Autodesk Inventor part; units mm, degrees
ref_plane "FOR_PIN_1_XY" through (0, 2, 0) normal (0, 1, 0) x (1, 0, 0)
ref_plane "FOR_PIN_1_YZ" through (0, 2, 0) normal (1, 0, 0) x (0, 0, -1)
ref_plane "FOR_PIN_1_ZX" through (0, 2, 0) normal (0, 0, -1) x (0, 1, 0)
sketch "Sketch_2" plane through (0, 0, 0) normal (0, 1, 0) x (-1, 0, 0)
  line L0 (1, -0.402) -> (1, 0.402)
  line L1 (1, 0.402) -> (0.7211, 1)
  line L2 (0.7211, 1) -> (-0.7211, 1)
  line L3 (-0.7211, 1) -> (-1, 0.402)
  line L4 (-1, 0.402) -> (-1, -0.402)
  line L5 (-1, -0.402) -> (-0.7211, -1)
  line L6 (-0.7211, -1) -> (0.7211, -1)
  line L7 (0.7211, -1) -> (1, -0.402)
extrude "Extrusion1" add sketch "Sketch_2" along normal blind 2
pattern_linear "Rectangular Pattern1" count 6 spacing 2 along (1, 0, 0) of "Extrusion1"
sketch "Sketch_6" plane through (-1, 0, 0) normal (1, 0, 0) x (0, 0, -1)
  line L0 (-0.75, 0.5) -> (-0.75, 0)
  line L1 (-0.75, 0) -> (0.75, 0)
  line L2 (0.75, 0) -> (0.75, 0.5)
  line L3 (0.75, 0.5) -> (-0.75, 0.5)
extrude "Extrusion2" cut sketch "Sketch_6" along normal blind 12
sketch "Sketch_4" plane through (0, 0, 0) normal (0, 1, 0) x (-1, 0, 0)
  line L0 (0.25, -0.25) -> (0.25, 0.25)
  line L1 (0.25, 0.25) -> (-0.25, 0.25)
  line L2 (-0.25, 0.25) -> (-0.25, -0.25)
  line L3 (-0.25, -0.25) -> (0.25, -0.25)
extrude "Extrusion3" cut sketch "Sketch_4" along normal blind 2
pattern_linear "Rectangular Pattern2" count 6 spacing 2 along (1, 0, 0) of "Extrusion3"
sketch "Sketch_9" plane through (0, 0, 0) normal (0, 0, 1) x (1, 0, 0)
  line L0 (-1.28, 0.5) -> (-1.28, 0)
  line L1 (-1.28, 0) -> (-0.72, 0)
  line L2 (-0.72, 0) -> (-0.72, 0.5)
  line L3 (-0.72, 0.5) -> (-1.28, 0.5)
extrude "Extrusion4" cut sketch "Sketch_9" along normal mid plane 2
pattern_linear "Rectangular Pattern3" count 7 spacing 2 along (1, 0, 0) of "Extrusion4"
ref_plane "FOR_PIN_1_XY" through (0, 2, 0) normal (0, 1, 0) x (1, 0, 0)
ref_plane "FOR_PIN_1_YZ" through (0, 2, 0) normal (1, 0, 0) x (0, 0, -1)
ref_plane "FOR_PIN_1_ZX" through (0, 2, 0) normal (0, 0, -1) x (0, 1, 0)
ref_plane "FOR_PIN_2_XY" through (2, 2, 0) normal (0, 1, 0) x (1, 0, 0)
ref_plane "FOR_PIN_2_YZ" through (2, 2, 0) normal (1, 0, 0) x (0, 0, -1)
ref_plane "FOR_PIN_2_ZX" through (2, 2, 0) normal (0, 0, -1) x (0, 1, 0)
ref_plane "FOR_PIN_3_XY" through (4, 2, 0) normal (0, 1, 0) x (1, 0, 0)
ref_plane "FOR_PIN_3_YZ" through (4, 2, 0) normal (1, 0, 0) x (0, 0, -1)
ref_plane "FOR_PIN_3_ZX" through (4, 2, 0) normal (0, 0, -1) x (0, 1, 0)
ref_plane "FOR_PIN_4_XY" through (6, 2, 0) normal (0, 1, 0) x (1, 0, 0)
ref_plane "FOR_PIN_4_YZ" through (6, 2, 0) normal (1, 0, 0) x (0, 0, -1)
ref_plane "FOR_PIN_4_ZX" through (6, 2, 0) normal (0, 0, -1) x (0, 1, 0)
ref_plane "FOR_PIN_5_XY" through (8, 2, 0) normal (0, 1, 0) x (1, 0, 0)
ref_plane "FOR_PIN_5_YZ" through (8, 2, 0) normal (1, 0, 0) x (0, 0, -1)
ref_plane "FOR_PIN_5_ZX" through (8, 2, 0) normal (0, 0, -1) x (0, 1, 0)
ref_plane "FOR_PIN_6_XY" through (10, 2, 0) normal (0, 1, 0) x (1, 0, 0)
ref_plane "FOR_PIN_6_YZ" through (10, 2, 0) normal (1, 0, 0) x (0, 0, -1)
ref_plane "FOR_PIN_6_ZX" through (10, 2, 0) normal (0, 0, -1) x (0, 1, 0)
ref_plane "IP_HOUSING_XY" through (-1, 0, 0) normal (0, 1, 0) x (1, 0, 0)
ref_plane "IP_HOUSING_YZ" through (-1, 0, 0) normal (1, 0, 0) x (0, 0, -1)
ref_plane "IP_HOUSING_ZX" through (-1, 0, 0) normal (0, 0, -1) x (0, 1, 0)
properties part number "BF021-06-A-B-0400-0280-N-G_H"
Geometry check sheet. Reference: the model listing, model coordinates, mm. Give positions to 0.01 mm unless a question says otherwise; leave off trailing zeros. Order: outer loops, then holes, each group sorted by start corner. A loop starts at its lowest first (then second) coordinate and runs counter-clockwise, first axis right, second up.
1. Sectioned sample at C-C (x = 2.5). Record the boundary of the cut face in (y, z).
Completed:
outline: (0, -1) - (2, -1) - (2, 1) - (0, 1) - (0, 0.75) - (0.5, 0.75) - (0.5, -0.75) - (0, -0.75) - close
2. Sectioned sample at A-A (x = 8). Record the boundary of the cut face in (y, z).
Completed:
outline: (0, -1) - (2, -1) - (2, -0.25) - (0.5, -0.25) - (0.5, -0.75) - (0, -0.75) - close; (0, 0.75) - (0.5, 0.75) - (0.5, 0.25) - (2, 0.25) - (2, 1) - (0, 1) - close
3. Scan lines: line 1 (Z direction, x = 6, y = 1.4); line 2 (Z direction, x = 4.5, y = 0.25); line 3 (X direction, y = 1.85, z = 0.65). Record each from-to range of solid material in increasing order.
Completed:
line 1: z = -1 to -0.25, 0.25 to 1
line 2: z = -1 to -0.75, 0.75 to 1
line 3: x = -0.88 to 0.88, 1.12 to 2.88, 3.12 to 4.88, 5.12 to 6.88, 7.12 to 8.88, 9.12 to 10.88
4. Sectioned sample at B-B (z = -0.05). Record the boundary of the cut face in (x, y), then the cut area to 3 significant figures.
Completed:
outline: (-1, 0.5) - (-0.25, 0.5) - (-0.25, 2) - (-1, 2) - close; (0.25, 0.5) - (1.75, 0.5) - (1.75, 2) - (0.25, 2) - close; (2.25, 0.5) - (3.75, 0.5) - (3.75, 2) - (2.25, 2) - close; (4.25, 0.5) - (5.75, 0.5) - (5.75, 2) - (4.25, 2) - close; (6.25, 0.5) - (7.75, 0.5) - (7.75, 2) - (6.25, 2) - close; (8.25, 0.5) - (9.75, 0.5) - (9.75, 2) - (8.25, 2) - close; (10.25, 0.5) - (11, 0.5) - (11, 2) - (10.25, 2) - close
area: 13.5 mm2
5. Sectioned sample at D-D (y = 0.65). State how many separate pieces and enclosed holes the cut face has, then the cut area to 3 significant figures.
Completed:
separate pieces: 1
enclosed holes: 6
area: 20.5 mm2
